Design review of the part built by this model. Coordinates are the model's own, in mm. A direction names the side the tool comes from. Give positions to 0.01 mm unless a question says otherwise; leave off trailing zeros. Write each loop counter-clockwise with the first axis right and the second up, starting at its lowest first coordinate (ties: lowest second). Pieces come first, ordered by that corner, then holes.
```python
from build123d import *

# Parameters (mm, degrees)
ESQUISSE1_W                  = 103
ESQUISSE1_H                  = 10
ENL_V_MAT_EXTRU_4_DEPTH      = 104.966340707
ENL_V_MAT_EXTRU_4_DEPTH_BACK = 104.966340707
ESQUISSE8_R                  = 5.983
ENL_V_START                  = 5
ESQUISSE9_W                  = 14
ESQUISSE9_H                  = 20
ENL_V_MAT_EXTRU_6_DEPTH      = 99.966340826


with BuildPart() as part:
    # Esquisse1 → Révolution1 (revolve)
    with BuildSketch(Plane.XY, mode=Mode.PRIVATE) as r_volution1_sk:
        with Locations((51.5, 5)):
            Rectangle(ESQUISSE1_W, ESQUISSE1_H)
    revolve(r_volution1_sk.sketch.rotate(Axis((0, 0, 0), (1, 0, 0)), 90), axis=Axis((0, 0, 0), (1, 0, 0)))

    # Esquisse8 → Enlèv. mat.-Extru.4 (cut, two sides: drawn at the far end of the back side and taken through both)
    with BuildSketch(Plane(origin=(0, 0, 0), x_dir=(1, 0, 0), z_dir=(0, 1, 0)).offset(-ENL_V_MAT_EXTRU_4_DEPTH_BACK)):
        with Locations(Location((14, 0, 0), (0, 0, 270))):
            Circle(ESQUISSE8_R)
        with Locations(Location((89, 0, 0), (0, 0, 270))):
            Circle(ESQUISSE8_R)
    extrude(amount=ENL_V_MAT_EXTRU_4_DEPTH + ENL_V_MAT_EXTRU_4_DEPTH_BACK, mode=Mode.SUBTRACT)

    # Esquisse9 → Enlèv. mat.-Extru.6 (cut, through all)
    with BuildSketch(Plane(origin=(0, 0, 0), x_dir=(1, 0, 0), z_dir=(0, 1, 0)).offset(ENL_V_START)):
        with Locations((14, 0)):
            Rectangle(ESQUISSE9_W, ESQUISSE9_H)
        with Locations((89, 0)):
            Rectangle(ESQUISSE9_W, ESQUISSE9_H)
    extrude(amount=ENL_V_MAT_EXTRU_6_DEPTH, mode=Mode.SUBTRACT)


solid = part.part
```
(1) Consider section D-D, the plane x = 26. Give the boundary of the cut face in (y, z), then the cut area to 3 significant figures.
Resolved:
outline: circle Ø20 at (0, 0)
area: 314 mm2
(2) Consider section A-A, the plane y = 6. Give the boundary of the cut face in (x, z), then the cut area to 3 significant figures.
Resolved:
outline: (0, -8) - (7, -8) - (7, 8) - (0, 8) - close; (21, -8) - (82, -8) - (82, 8) - (21, 8) - close; (96, -8) - (103, -8) - (103, 8) - (96, 8) - close
area: 1,200 mm2
(3) Clearance check with flat-ended pins moving along their axes: P1, Ø1.5, axis at x = 35.5, y = -2, coming from the +Z side; P2, Ø11, axis at x = 90, z = 1.5, coming from the +Y side; P3, Ø4, axis at x = 27, z = 3, coming from the +Y side. State where each tip first meets the part, or that it passes through.
Resolved:
P1: stops at z = 9.92
P2: stops at y = 5
P3: stops at y = 9.95
(4) To check wall thickness, follow L1, parallel to X at y = -4, z = 0; L2, parallel to X at y = -8.25, z = -1.25; L3, parallel to Y at x = 61, z = 5. State the ranges of each line that lie inside material, in increasing order.
Resolved:
L1: x = 0 to 8.02, 19.98 to 83.02, 94.98 to 103
L2: x = 0 to 8.15, 19.85 to 83.15, 94.85 to 103
L3: y = -8.66 to 8.66
(5) Consider section C-C, the plane y = -6. Give the boundary of the cut face in (x, z), then the cut area to 3 significant figures.
Resolved:
outline: (0, -8) - (103, -8) - (103, 8) - (0, 8) - close; hole circle Ø11.97 at (14, 0); hole circle Ø11.97 at (89, 0)
area: 1,420 mm2
(6) Tool access review of faces 4 (the face through (21, 7, 0)), 5 (the face through (15.797, -2.613, 5.707)): name each direction out of +Z, -Z, +X, -X, +Y, -Y from which nothing blocks a thin tool from reaching the whole face with its end or side.
Resolved:
face 4: +Z, -Z, +Y
face 5: +Y, -Y
(7) Mouldability with a two-part tool opening along X and no side actions: class faces 1 (the face through (12, 5, -6)), 2 (the face through (103, 0, 0)), 3 (the face through (0, 0, 0)) as pulls with the +X half, pulls with the -X half, needs draft (parallel to the pull), parting line crosses it, or undercut.
Resolved:
face 1: undercut
face 2: pulls with the +X half
face 3: pulls with the -X half
(8) Consider section B-B, the plane z = 0. Give the boundary of the cut face in (x, y).
Resolved:
outline: (0, -10) - (8.02, -10) - (8.02, 5) - (7, 5) - (7, 10) - (0, 10) - close; (19.98, -10) - (83.02, -10) - (83.02, 5) - (82, 5) - (82, 10) - (21, 10) - (21, 5) - (19.98, 5) - close; (94.98, -10) - (103, -10) - (103, 10) - (96, 10) - (96, 5) - (94.98, 5) - close
